Input: dimensioned drawing with shaded views. Units: mm. Origin: part minimum x, y, z. A direction names the side the tool comes from. Round coordinates to 2 decimals unless told otherwise and drop trailing zeros. Loops run counter-clockwise (first coordinate to the right, second up) from the corner with the lowest first, then second, coordinate; pieces in that order, holes last. Notation, with made-up numbers: (-33, 66.5) - (-20, 66.5) arc R17 ccw to (-20, 84.5) - close; hole circle Ø11 at (-39.75, -9). An arc over 180 degrees is marked (long way). One line per question, with ' | ' between items.
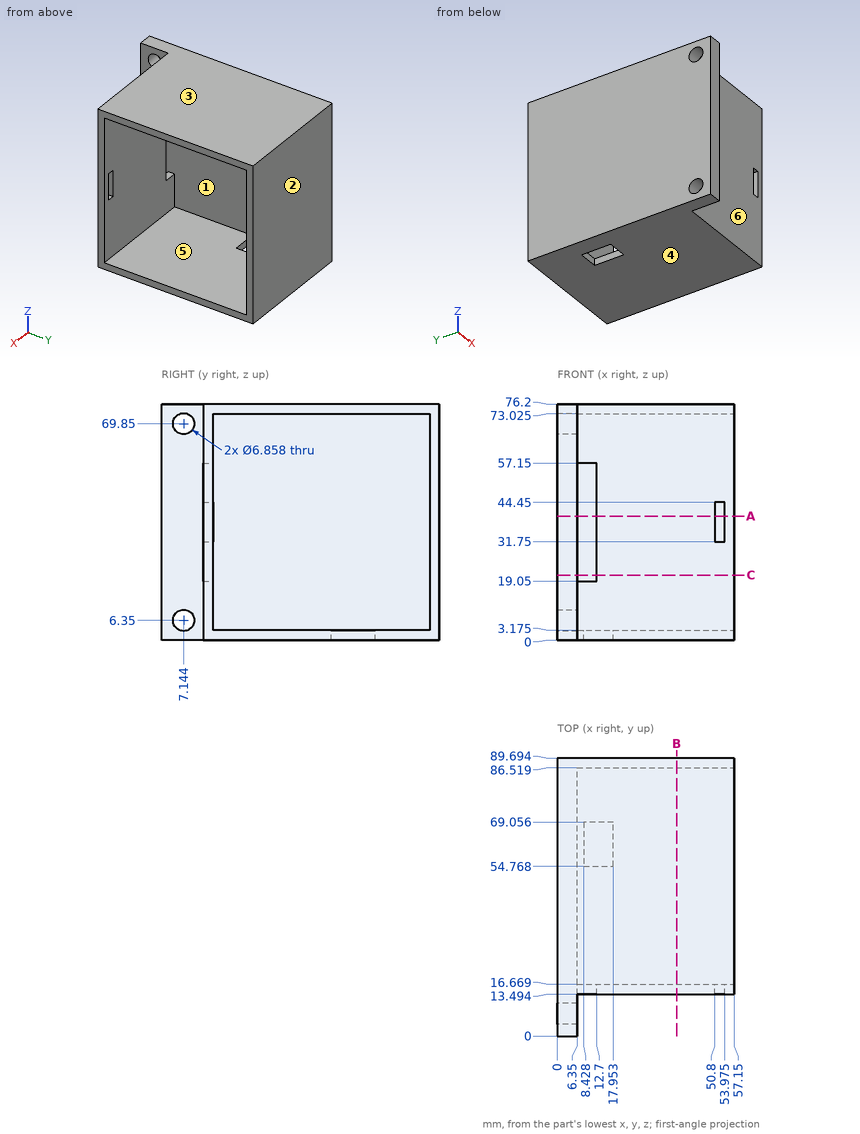
1. Material intervals for probe 1 along Z at (x, y) = (40, 30) (1 decimal); probe 2 along Y at (x, z) = (27.5, 35); probe 3 along Y at (x, z) = (4.75, 69.85) (1 decimal), sorted ascending.
Worked out:
probe 1: z = 0 to 3.2, 73 to 76.2 | probe 2: y = 13.49 to 16.67, 86.52 to 89.69 | probe 3: y = 0 to 3.7, 10.6 to 89.7
2. Section query C-C, the plane z = 21. Return loops of the section in (x, y), plus the area to 3 significant figures.
Worked out:
outline: (0, 0) - (6.35, 0) - (6.35, 86.52) - (57.15, 86.52) - (57.15, 89.69) - (0, 89.69) - close; (12.7, 13.49) - (57.15, 13.49) - (57.15, 16.67) - (12.7, 16.67) - close | area: 872 mm2
3. Section query B-B, the plane x = 38.5. Return loops of the section in (y, z) (1 decimal).
Worked out:
outline: (13.5, 0) - (89.7, 0) - (89.7, 76.2) - (13.5, 76.2) - close; hole (16.7, 3.2) - (86.5, 3.2) - (86.5, 73) - (16.7, 73) - close
4. Section query A-A, the plane z = 40. Give the number of separate pieces and of enclosed holes in the cut face, plus the area to 3 significant figures.
Worked out:
separate pieces: 3 | enclosed holes: 0 | area: 862 mm2
5. Mould query, pull axis Z, two halves, no side actions, for the marked faces 1, 2 and 3. Classes: released by +Z, released by -Z, zero draft, split by the parting line, or undercut.
Worked out:
face 1: undercut | face 2: zero draft | face 3: released by +Z
6. Access query for the marked faces 4, 5 and 6. Directions: +Z, -Z, +X, -X, +Y, -Y. A direction counts if a zero-diameter tool reaches every point of the face in a straight line with its end or side. Return the directions, or none.
Worked out:
face 4: -Z, +X, -X, +Y, -Y | face 5: +X | face 6: +Z, -Z, +X, -Y
7. Contact query for flat-ended pins moving along their axis: P1, Ø3.5, axis at x = 11.5, z = 1, coming from the -Y side; P2, Ø15, axis at x = 42, y = 66.5, coming from the -Z side; P3, Ø8, axis at y = 73.5, z = 13.5, coming from the +X side. Output: stop coordinate, or through.
Worked out:
P1: stops at y = 13.49 | P2: stops at z = 0 | P3: stops at x = 6.35
